Geometry check sheet. Reference: the model listing, model coordinates, mm. A direction names the side the tool comes from. Coordinates: 2 decimals unless noted, no trailing zeros. Write each loop counter-clockwise with the first axis right and the second up, starting at its lowest first coordinate (ties: lowest second). Pieces come first, ordered by that corner, then holes. Notation, with made-up numbers: (41, 34.25) -> (56, 34.25) arc R3 ccw to (56, 38.25) -> close; hole circle Ø5 at (26.25, 81.25). An arc over 180 degrees is marked (long way). One line per question, with ' | ' between items.
Autodesk Inventor part; units mm, degrees
ref_plane "YZ Plane" through (0, 0, 0) normal (1, 0, 0) x (0, 1, 0)
ref_plane "XZ Plane" through (0, 0, 0) normal (0, 1, 0) x (-1, 0, 0)
ref_plane "XY Plane" through (0, 0, 0) normal (0, 0, 1) x (1, 0, 0)
sketch "Эскиз1" plane through (0, 0, 0) normal (0, 1, 0) x (-1, 0, 0)
  circle A0 centre (0, 0) radius 10
  circle A1 centre (0, 0) radius 1.5
  circle A2 centre (7, 0) radius 1.5
  circle A3 centre (0, -7) radius 1.5
  circle A4 centre (-7, 0) radius 1.5
  circle A5 centre (0, 7) radius 1.5
  dimension "d0" = 20
  dimension "d1" = 3
  dimension "d2" = 3
  dimension "d3" = 3
  dimension "d4" = 3
  dimension "d5" = 3
  dimension "d6" = 7
  dimension "d7" = 7
  dimension "d8" = 7
  dimension "d9" = 7
extrude "Выдавливание1" add sketch "Эскиз1" along normal blind 2
sketch "Эскиз2" plane through (0, 0, 0) normal (0, -1, 0) x (1, 0, 0)
  circle A0 centre (0, 0) radius 1.5
  circle A1 centre (0, 0) radius 3
  circle A2 centre (0, 0) radius 4.5
  dimension "d12" = 6
  dimension "d13" = 9
extrude "Выдавливание2" add sketch "Эскиз2" along normal blind 2.5 contours A2
sketch "Эскиз3" plane through (0, 0, 0) normal (0, -1, 0) x (1, 0, 0)
  circle A0 centre (0, 0) radius 1.5
  circle A1 centre (0, 0) radius 3
extrude "Выдавливание3" cut sketch "Эскиз3" against normal blind 1
properties part number "MG996R_nozzle"
1. Cross-section at D-D on x = 8.25. Record the boundary of the cut face in (y, z), and give its area (3 significant figures).
Worked answers:
outline: (0, -5.65) -> (2, -5.65) -> (2, -0.83) -> (0, -0.83) -> close; (0, 0.83) -> (2, 0.83) -> (2, 5.65) -> (0, 5.65) -> close | area: 19.3 mm²
2. Cross-section at B-B on z = 0. Record the boundary of the cut face in (x, y).
Worked answers:
outline: (-10, 0) -> (-8.5, 0) -> (-8.5, 2) -> (-10, 2) -> close; (-5.5, 0) -> (-4.5, 0) -> (-4.5, -2.5) -> (-3, -2.5) -> (-3, 1) -> (-1.5, 1) -> (-1.5, 2) -> (-5.5, 2) -> close; (1.5, 1) -> (3, 1) -> (3, -2.5) -> (4.5, -2.5) -> (4.5, 0) -> (5.5, 0) -> (5.5, 2) -> (1.5, 2) -> close; (8.5, 0) -> (10, 0) -> (10, 2) -> (8.5, 2) -> close
3. Cross-section at C-C on y = 1.6. Record the boundary of the cut face in (x, z), and give its area (3 significant figures).
Worked answers:
outline: circle Ø20 at (0, 0); hole circle Ø3 at (-7, 0); hole circle Ø3 at (0, -7); hole circle Ø3 at (0, 0); hole circle Ø3 at (0, 7); hole circle Ø3 at (7, 0) | area: 279 mm²
4. Cross-section at A-A on x = 0. Record the boundary of the cut face in (y, z).
Worked answers:
outline: (-2.5, -4.5) -> (0, -4.5) -> (0, -5.5) -> (2, -5.5) -> (2, -1.5) -> (1, -1.5) -> (1, -3) -> (-2.5, -3) -> close; (-2.5, 3) -> (1, 3) -> (1, 1.5) -> (2, 1.5) -> (2, 5.5) -> (0, 5.5) -> (0, 4.5) -> (-2.5, 4.5) -> close; (0, -10) -> (2, -10) -> (2, -8.5) -> (0, -8.5) -> close; (0, 8.5) -> (2, 8.5) -> (2, 10) -> (0, 10) -> close
5. Material ranges on line 1 (Z direction, x = 0, y = 1.3); line 2 (Z direction, x = 0, y = 0.1); line 3 (X direction, y = 1.8, z = 0.5), recorded low to high. Write a range as from..to.
Worked answers:
line 1: -10..-8.5, -5.5..-1.5, 1.5..5.5, 8.5..10 | line 2: -10..-8.5, -5.5..-3, 3..5.5, 8.5..10 | line 3: -9.99..-8.41, -5.59..-1.41, 1.41..5.59, 8.41..9.99
6. Mould release check, pull along Z, two halves, no side actions. Record for faces 1 (the face through (-3, -1, 0)), 2 (the face through (2.17, 0.99, 9.76)), 3 (the face through (-2, 2, 0)): released by +Z, released by -Z, zero draft, split by the parting line, or undercut.
Worked answers:
face 1: undercut | face 2: split by the parting line | face 3: zero draft
7. Go/stop test with flat-tipped pins: P1, Ø1, axis at x = -0.5, z = 1, coming from the -Y side; P2, Ø3.5, axis at x = 0, z = -7, coming from the -Y side. Record where each tip stops, or that it passes through.
Worked answers:
P1: y = 1 | P2: y = 0
8. Tool access check on faces 4 (the face through (0.325, 0.986, 8.464)), 5 (the face through (-0.59, -1.23, -4.46)). Record the directions out of +Z, -Z, +X, -X, +Y, -Y that give a thin tool (end or side, any length) a straight path to the whole face; none if there is none.
Worked answers:
face 4: +Y, -Y | face 5: -Y
